The listing builds one solid part. Answer for the finished solid, in the listing's coordinates (mm). Face numbers are marked on the shaded views. A direction names the side the tool comes from. Coordinates: 2 decimals unless noted, no trailing zeros. Order: outer loops, then holes, each group sorted by start corner. A loop starts at its lowest first (then second) coordinate and runs counter-clockwise, first axis right, second up.
Autodesk Inventor part; units mm, degrees
ref_plane "YZ Plane" through (0, 0, 0) normal (1, 0, 0) x (0, 1, 0)
ref_plane "XZ Plane" through (0, 0, 0) normal (0, 1, 0) x (-1, 0, 0)
sketch "Top" plane through (0, 0, 0) normal (0, 0, 1) x (1, 0, 0)
  line L0 (0, 8) -> (0, 0)
  line L1 (0, 0) -> (16, 0)
  line L2 (16, 0) -> (16, 8)
  line L3 (0, 8) -> (16, 8)
  point P0 (8, 0)
  dimension "d0" = 16
  dimension "d1" = 8
  dimension "d2" = 8
extrude "Extrusion5" add sketch "Top" against normal blind 8
sketch "Sketch4" plane through (0, 0, 0) normal (0, 0, 1) x (1, 0, 0)
  line L0 (0, 0) -> (0, 8)
  line L1 (16, 8) -> (16, 0)
  line L2 (0, 8) -> (16, 8)
  line L3 (16, 8) -> (16, 0)
  line L4 (16, 0) -> (0, 0)
  line L5 (0, 0) -> (0, 8)
  circle A0 centre (4, 4) radius 2.4
  circle A1 centre (12, 4) radius 2.4
  dimension "d29" = 4.8
  dimension "d30" = 4.8
  dimension "d31" = 4
  dimension "d32" = 4
  dimension "d33" = 8
  dimension "d34" = 4
extrude "Extrusion6" add sketch "Sketch4" along normal blind 1.8 contours A0 | A1
sketch "Sketch5" plane through (0, 0, -8) normal (0, 0, -1) x (-1, 0, 0)
  line L0 (-14.9, 6.9) -> (-1.1, 6.9)
  line L1 (-1.1, 6.9) -> (-1.1, 1.1)
  line L2 (-1.1, 1.1) -> (-14.9, 1.1)
  line L3 (-14.9, 1.1) -> (-14.9, 6.9)
  line L4 (0, 8) -> (-16, 8)
  line L5 (-16, 8) -> (-16, 0)
  line L6 (-16, 0) -> (0, 0)
  line L7 (0, 0) -> (0, 8)
  dimension "d37" = 1.1
  dimension "d38" = 1.1
  dimension "d39" = 1.1
  dimension "d40" = 1.1
extrude "Extrusion7" cut sketch "Sketch5" against normal blind 1.2 contours L0 L1 L2 L3
sketch "Sketch6" plane through (0, 0, -6.8) normal (0, 0, -1) x (-1, 0, 0)
  line L0 (-14.9, 1.1) -> (-14.9, 6.9)
  line L1 (-14.9, 4.2225) -> (-1.1, 4.2225)
  line L2 (-1.1, 6.9) -> (-1.1, 1.1)
  circle A0 centre (-8, 4.2225) radius 2
  line L3 (-16, 8) -> (-16, 0)
  line L4 (-1.1, 1.1) -> (-14.9, 1.1)
  point P0 (0, 0)
  dimension "d43" = 8
  dimension "d44" = 4
  dimension "d45" = 3.1225
extrude "Extrusion8" add sketch "Sketch6" along normal blind 1.2 contours A0 L1 | L1 A0
sketch "Sketch8" plane through (0, 8, 0) normal (0, 1, 0) x (1, 0, 0)
  line L0 (16, 0) -> (16, 8)
  line L1 (16, 4) -> (0, 4)
  line L2 (0, 0) -> (0, 8)
  point P0 (8, 4)
hole "Hole2" at (8, 8, -4) direction (0, -1, 0) diameter 4 depth 8 tip angle 118
properties part number "bricks"
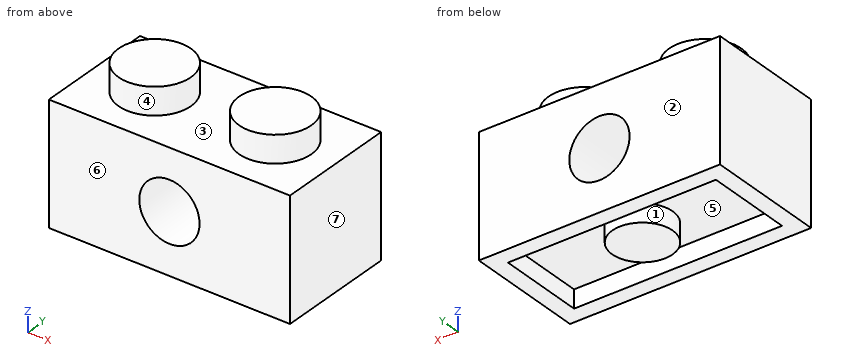
(1) For the marked faces 1, 2 and 3, determine the directions among +Z, -Z, +X, -X, +Y, -Y from which every point of the face is accessible in a straight line to the end or side of a thin tool.
(2) The mould has two halves that part along X. Classify the marked faces 4, 5, 6 and 7: released by +X, released by -X, zero draft, split by the parting line, or undercut.
(3) Find section A-A (z = -4). Write down the section's boundary in (x, y).
(4) Find section C-C (y = 3.5). Write down the section's boundary in (x, z), and give its area (3 significant figures).
(5) Find section B-B (x = 8). Write down the section's boundary in (y, z), and give its area (3 significant figures).
(6) Consider line 1 (Y direction, x = 14.75, z = -7); line 2 (X direction, y = 2.5, z = -4); line 3 (Y direction, x = 9.25, z = -7). Determine where each line is inside the solid, lowest interval first.
(7) Each of these flat-tipped pins is pushed along its axis until it touches: pin 1 Ø0.6 at (y, z) = (4, -7.5) entering from -X; pin 2 Ø3 at (x, z) = (8, -4) entering from -Y. Where does it stop, or does it pass through?
(8) Find section D-D (x = 12). Write down the section's boundary in (y, z).
Findings below:
1. face 1: -Z
1. face 2: +Z, -Z, +X, -X, +Y
1. face 3: +Z
2. face 4: undercut
2. face 5: undercut
2. face 6: zero draft
2. face 7: released by +X
3. outline: (0, 0) - (6, 0) - (6, 8) - (0, 8) - close; (10, 0) - (16, 0) - (16, 8) - (10, 8) - close
4. outline: (0, -8) - (1.1, -8) - (1.1, -6.8) - (6.14, -6.8) - (6.14, -8) - (9.86, -8) - (9.86, -6.8) - (14.9, -6.8) - (14.9, -8) - (16, -8) - (16, 0) - (14.35, 0) - (14.35, 1.8) - (9.65, 1.8) - (9.65, 0) - (6.35, 0) - (6.35, 1.8) - (1.65, 1.8) - (1.65, 0) - (0, 0) - close; hole circle Ø4 at (8, -4)
4. area: 120 mm2
5. outline: (0, -8) - (1.1, -8) - (1.1, -6.8) - (2.22, -6.8) - (2.22, -8) - (6.22, -8) - (6.22, -6.8) - (6.9, -6.8) - (6.9, -8) - (8, -8) - (8, -6) - (0, -6) - close; (0, -2) - (8, -2) - (8, 0) - (0, 0) - close
5. area: 29.8 mm2
6. line 1: y = 0 to 1.1, 6.9 to 8
6. line 2: x = 0 to 6, 10 to 16
6. line 3: y = 0 to 1.1, 2.66 to 5.78, 6.9 to 8
7. pin 1: stops at x = 0
7. pin 2: passes through
8. outline: (0, -8) - (1.1, -8) - (1.1, -6.8) - (6.9, -6.8) - (6.9, -8) - (8, -8) - (8, 0) - (6.4, 0) - (6.4, 1.8) - (1.6, 1.8) - (1.6, 0) - (0, 0) - close
